Read the model definition and answer for the solid it produces. Units are mm, in the model's axes. Face numbers are marked on the shaded views. A direction names the side the tool comes from. Coordinates: 2 decimals unless noted, no trailing zeros. Loops run counter-clockwise (first coordinate to the right, second up) from the corner with the lowest first, then second, coordinate; pieces in that order, holes last. Notation, with made-up numbers: M 25.5,4.25 L 64.5,4.25 A22 cw 64.5,37.25 Z; hole C 66,-32.75 d4. An arc over 180 degrees is marked long. Use one line per item in the form item = value. Start each with the question number.
1. A tool of negligible diameter and unlimited length cuts with its end or side. For the marked faces 4, 5 and 6, from which of +Z, -Z, +X, -X, +Y, -Y can it reach the whole face along a straight path? Write none if from no direction.
2. The part is cut by section A-A (y = 11). Give the vertices of the cut face in (x, z), plus the area to 3 significant figures.
3. Find the intervals of material crossed by probe 1 along Y at (x, z) = (16, 5.5); probe 2 along Y at (x, z) = (-11, 6); probe 3 along X at (y, z) = (16.5, 2.5), in increasing order. Write a range as [from, to].
4. The part is cut by section B-B (x = 12). Give the vertices of the cut face in (y, z).
5. The part is cut by section D-D (x = -7). Give the vertices of the cut face in (y, z), plus the area to 3 significant figures.
6. The part is cut by section C-C (z = 6.25). Give the vertices of the cut face in (x, y), plus the area to 3 significant figures.
7. A flat-ended cylindrical pin translates along its axis: pin 1 (3 mm diameter, centred on x = -0.5, z = 6, fed in from -Y). Find the tip coordinate at first contact, or state that the pin passes through.
8. For a pull along X with two mould halves and no side action, classify the marked faces 1, 2 and 3 as released by +X, released by -X, zero draft, split by the parting line, or undercut.
from build123d import *

# Parameters (mm, degrees)
F1_DEPTH = 10


with BuildPart() as f1:
    # F0 (on Top) → F1 (new body)
    with BuildSketch(Plane.XY):
        Polygon((-10, 20), (-30, 20), (-30, -20), (-10, -20), (-10, -10), (-20, -10), (-20, 0), (-20, 10), (-10, 10), align=None)
        Polygon((30, 20), (0, 20), (0, 10), (10, 10), (20, 10), (20, -10), (10, -10), (10, -20), (30, -20), align=None)
        Polygon((0, 10), (-10, 10), (-20, 10), (-20, 0), (10, 0), (10, 10), align=None)
    extrude(amount=F1_DEPTH)


solid = f1.part
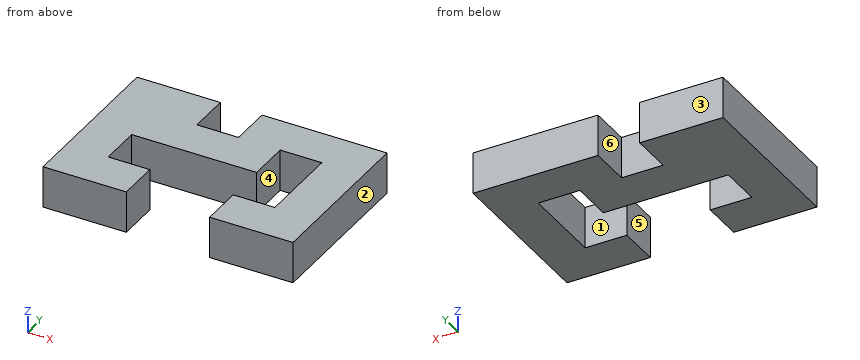
Computed values:
q1.face_4 = +Z, -Z
q1.face_5 = +Z, -Z, -Y
q1.face_6 = +Z, -Z, +Y
q2.outline = M -30,0 L -10,0 L -10,10 L -30,10 Z; M 0,0 L 30,0 L 30,10 L 0,10 Z
q2.area = 500 mm²
q3.probe_1 = [-20, -10], [10, 20]
q3.probe_2 = [-20, -10], [0, 20]
q3.probe_3 = [-30, -10], [0, 30]
q4.outline = M -20,0 L -10,0 L -10,10 L -20,10 Z; M 10,0 L 20,0 L 20,10 L 10,10 Z
q5.outline = M 0,0 L 10,0 L 10,10 L 0,10 Z
q5.area = 100 mm²
q6.outline = M -30,-20 L -10,-20 L -10,-10 L -20,-10 L -20,0 L 10,0 L 10,10 L 20,10 L 20,-10 L 10,-10 L 10,-20 L 30,-20 L 30,20 L 0,20 L 0,10 L -10,10 L -10,20 L -30,20 Z
q6.area = 1,600 mm²
q7.pin_1 = 0
q8.face_1 = undercut
q8.face_2 = released by +X
q8.face_3 = zero draft
